CAD build for the part. Positions are in the model's coordinates, mm. A direction names the side the tool comes from. Give positions to 0.01 mm unless a question says otherwise; leave off trailing zeros. Write each loop counter-clockwise with the first axis right and the second up, starting at its lowest first coordinate (ties: lowest second). Pieces come first, ordered by that corner, then holes. Notation, with made-up numbers: (-27, 69.5) - (-19, 69.5) arc R20 ccw to (-19, 108.5) - close; hole circle Ø10 at (-18, -11). An arc over 180 degrees is marked (long way). Answer as a JSON object with one key per item and string values.
from build123d import *

# Parameters (mm, degrees)
F1_DEPTH = 25.4
F3_DEPTH = 12.780771


with BuildPart() as f1:
    # F0 (on Top) → F1 (new body)
    with BuildSketch(Plane.XY):
        Polygon((16.532764, 0), (0, 76.285757), (-75.997785, 76.285757), (-92.152342, 0), (-75.602874, -76.248273), (0, -76.248273), align=None)
    extrude(amount=F1_DEPTH)

    # F2 (on face) → F3 (join)
    with BuildSketch(Plane.XY.offset(25.4)):
        Polygon((0, 0), (0, -76.248273), (16.532764, 0), (0, 76.285757), align=None)
    extrude(amount=F3_DEPTH)


solid = f1.part
(1) Saw through at D-D, the plane z = 33.5. Give the cut face in (x, y), and give its area (3 significant figures).
Answer key:
{"outline": "(0, -76.25) - (16.53, 0) - (0, 76.29) - close", "area": "1,260 mm²"}
(2) Flat gauge pins, fed straight in: P1, Ø14, axis at y = -36, z = 32.5, coming from the -X side; P2, Ø2, axis at y = 42.5, z = 20, coming from the -X side; P3, Ø4, axis at x = -18, y = 23, coming from the -Z side; P4, Ø2, axis at y = 28, z = 14, coming from the -X side. Where does each tip first touch, or does it go through?
Answer key:
{"P1": "stops at x = 0", "P2": "stops at x = -83.36", "P3": "stops at z = 0", "P4": "stops at x = -86.43"}
(3) Saw through at B-B, the plane y = 30. Give the cut face in (x, z), and give its area (3 significant figures).
Answer key:
{"outline": "(-85.8, 0) - (10.03, 0) - (10.03, 38.18) - (0, 38.18) - (0, 25.4) - (-85.8, 25.4) - close", "area": "2,560 mm²"}
(4) Probe L1, parallel to Z at x = -37, y = 62.5; L2, parallel to X at y = -68, z = 7; L3, parallel to X at y = -12.5, z = 4. List the from-to ranges inside material, lowest first. Write a range as [from, to].
Answer key:
{"L1": "z = [0, 25.4]", "L2": "x = [-77.39, 1.79]", "L3": "x = [-89.44, 13.82]"}
(5) Saw through at A-A, the plane z = 8. Give the cut face in (x, y).
Answer key:
{"outline": "(-92.15, 0) - (-75.6, -76.25) - (0, -76.25) - (16.53, 0) - (0, 76.29) - (-76, 76.29) - close"}
(6) 3-axis set-ups, long thin cutter, end or side, ignore diameter. For faces 1 (the face through (-38, -76.248, 13)), 2 (the face through (0, 1, 32)): which of +Z, -Z, +X, -X, +Y, -Y reach the whole face in a straight line?
Answer key:
{"face 1": "+Z, -Z, +X, -X, -Y", "face 2": "+Z, -X, +Y, -Y"}
(7) Saw through at C-C, the plane x = -82.5. Give the cut face in (y, z).
Answer key:
{"outline": "(-44.47, 0) - (45.58, 0) - (45.58, 25.4) - (-44.47, 25.4) - close"}
